from build123d import *

# Parameters (mm, degrees)
SKETCH2_W                 = 250
SKETCH2_H                 = 150
BOSS_EXTRUDE1_DEPTH       = 4
BOSS_EXTRUDE2_DEPTH       = 4
SKETCH4_R                 = 4
CUT_EXTRUDE1_DEPTH        = 5
SKETCH5_R                 = 14
SKETCH5_R_2               = 11
BOSS_EXTRUDE3_DEPTH       = 7
MIRROR2_COPY_1_DEPTH      = 4
MIRROR2_COPY_2_SKETCH_R   = 4
MIRROR2_COPY_2_DEPTH      = 5
MIRROR2_COPY_3_SKETCH_R   = 14
MIRROR2_COPY_3_SKETCH_R_2 = 11
MIRROR2_COPY_3_DEPTH      = 7


with BuildPart() as part:
    # Sketch2 → Boss-Extrude1 (new body)
    with BuildSketch(Plane(origin=(0, 0, 0), x_dir=(1, 0, 0), z_dir=(0, 1, 0))):
        Rectangle(SKETCH2_W, SKETCH2_H)
    extrude(amount=BOSS_EXTRUDE1_DEPTH)

    # Sketch3 → Boss-Extrude2 (add)
    with BuildSketch(Plane(origin=(0, 4, 0), x_dir=(1, 0, 0), z_dir=(0, 1, 0))):
        Polygon((-103.786796564, 96.213203436), (-82.573593129, 75), (-125, 75), (-125, 32.573593129), (-146.213203436, 53.786796564), (-146.213203436, 96.213203436), align=None)
    boss_extrude2 = extrude(amount=-BOSS_EXTRUDE2_DEPTH)

    # Sketch4 → Cut-Extrude1 (cut, through all)
    with BuildSketch(Plane(origin=(0, 4, 0), x_dir=(1, 0, 0), z_dir=(0, 1, 0))):
        with Locations((-125, 75)):
            Circle(SKETCH4_R)
    cut_extrude1 = extrude(amount=-CUT_EXTRUDE1_DEPTH, mode=Mode.SUBTRACT)

    # Sketch5 → Boss-Extrude3 (add)
    with BuildSketch(Plane(origin=(0, 4, 0), x_dir=(1, 0, 0), z_dir=(0, 1, 0))):
        with Locations((-125, 75)):
            Circle(SKETCH5_R)
        with Locations((-125, 75)):
            Circle(SKETCH5_R_2, mode=Mode.SUBTRACT)
    boss_extrude3 = extrude(amount=BOSS_EXTRUDE3_DEPTH)

    # Mirror1: Boss-Extrude2, Cut-Extrude1, Boss-Extrude3 across plane
    add(boss_extrude2.mirror(Plane(origin=(0, 0, 0), x_dir=(0, 0, 1), z_dir=(1, 0, 0))))
    add(cut_extrude1.mirror(Plane(origin=(0, 0, 0), x_dir=(0, 0, 1), z_dir=(1, 0, 0))), mode=Mode.SUBTRACT)
    add(boss_extrude3.mirror(Plane(origin=(0, 0, 0), x_dir=(0, 0, 1), z_dir=(1, 0, 0))))

    # Mirror2: Boss-Extrude2, Cut-Extrude1, Boss-Extrude3 across plane
    add(boss_extrude2.mirror(Plane.XY))
    add(cut_extrude1.mirror(Plane.XY), mode=Mode.SUBTRACT)
    add(boss_extrude3.mirror(Plane.XY))

    # Mirror2 copy 1 sketch → Mirror2 copy 1 (add)
    with BuildSketch(Plane(origin=(0, 4, 0), x_dir=(-1, 0, 0), z_dir=(0, 1, 0))):
        Polygon((-103.786796564, 96.213203436), (-82.573593129, 75), (-125, 75), (-125, 32.573593129), (-146.213203436, 53.786796564), (-146.213203436, 96.213203436), align=None)
    extrude(amount=-MIRROR2_COPY_1_DEPTH)

    # Mirror2 copy 2 sketch → Mirror2 copy 2 (cut, through all)
    with BuildSketch(Plane(origin=(0, 4, 0), x_dir=(-1, 0, 0), z_dir=(0, 1, 0))):
        with Locations((-125, 75)):
            Circle(MIRROR2_COPY_2_SKETCH_R)
    extrude(amount=-MIRROR2_COPY_2_DEPTH, mode=Mode.SUBTRACT)

    # Mirror2 copy 3 sketch → Mirror2 copy 3 (add)
    with BuildSketch(Plane(origin=(0, 4, 0), x_dir=(-1, 0, 0), z_dir=(0, 1, 0))):
        with Locations((-125, 75)):
            Circle(MIRROR2_COPY_3_SKETCH_R)
        with Locations((-125, 75)):
            Circle(MIRROR2_COPY_3_SKETCH_R_2, mode=Mode.SUBTRACT)
    extrude(amount=MIRROR2_COPY_3_DEPTH)


solid = part.part
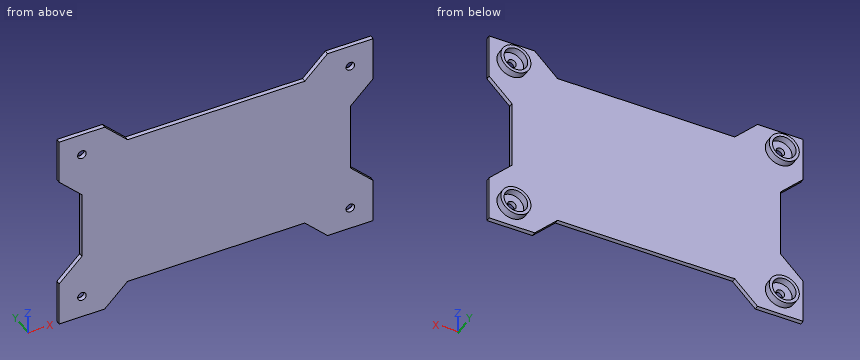
Design review of the part built by this model. Coordinates are the model's own, in mm. Coordinates: 2 decimals unless noted, no trailing zeros. Order: outer loops, then holes, each group sorted by start corner. A loop starts at its lowest first (then second) coordinate and runs counter-clockwise, first axis right, second up.
Item 1: Take a section at A-A, the plane y = 8. Write out the cut boundary in (x, z).
Item 2: Take a section at B-B, the plane x = 18. Write out the cut boundary in (y, z).
Item 3: For pin 1 Ø6 at (y, z) = (2.5, -32) entering from +X; pin 2 Ø2 at (x, y) = (-29, 2.5) entering from +Z; pin 3 Ø4.5 at (x, y) = (-10.5, 2) entering from -Z, all flat-tipped, find the tip position at first contact; note any pin that passes through.
Item 4: Take a section at C-C, the plane z = -14. Write out the cut boundary in (x, y), then the cut area to 3 significant figures.
Item 5: For line 1 (Z direction, x = 125, y = 7); line 2 (X direction, y = 6, z = -69); line 3 (Z direction, x = 117.5, y = 5), list the stretches that pass through material, from the lowest coordinate up.
The answers:
1. outline: circle Ø28 at (-125, -75); circle Ø28 at (-125, 75); circle Ø28 at (125, -75); circle Ø28 at (125, 75); hole circle Ø22 at (-125, -75); hole circle Ø22 at (-125, 75); hole circle Ø22 at (125, -75); hole circle Ø22 at (125, 75)
2. outline: (0, -75) - (4, -75) - (4, 75) - (0, 75) - close
3. pin 1: stops at x = 127.43
3. pin 2: stops at z = 75
3. pin 3: stops at z = -75
4. outline: (-125, 0) - (125, 0) - (125, 4) - (-125, 4) - close
4. area: 1,000 mm2
5. line 1: z = -89 to -86, -64 to -61, 61 to 64, 86 to 89
5. line 2: x = -137.65 to -134.22, -115.78 to -112.35, 112.35 to 115.78, 134.22 to 137.65
5. line 3: z = -86.82 to -83.05, -66.95 to -63.18, 63.18 to 66.95, 83.05 to 86.82
